```python
from build123d import *

# Parameters (mm, degrees)
EXTRUDE_THIN1_DEPTH = 165.1


with BuildPart() as part:
    # Sketch2 → Extrude-Thin1 (new body, symmetric)
    with BuildSketch(Plane(origin=(0, 0, 0), x_dir=(0, 0, -1), z_dir=(1, 0, 0))):
        with BuildLine():
            ThreePointArc((-60.240298086, -174.5682791), (-34.255387925, -150.550644745), (-24.65, -116.494825288))
            Line((-24.65, -116.494825288), (-24.65, -25.4))
            ThreePointArc((-24.65, -25.4), (-17.430182156, -7.969817844), (0, -0.75))
            Line((0, -0.75), (76.2, -0.75))
            Line((76.2, -0.75), (76.2, 0.75))
            Line((76.2, 0.75), (0, 0.75))
            ThreePointArc((0, 0.75), (-18.490842328, -6.909157672), (-26.15, -25.4))
            Line((-26.15, -25.4), (-26.15, -116.494825288))
            ThreePointArc((-26.15, -116.494825288), (-35.534320309, -149.766851432), (-60.921188809, -173.2317209))
            Line((-60.921188809, -173.2317209), (-60.240298086, -174.5682791))
        make_face()
    extrude(amount=EXTRUDE_THIN1_DEPTH, both=True)


solid = part.part
```
Design review of the part built by this model. Coordinates are the model's own, in mm. A direction names the side the tool comes from. Give positions to 0.01 mm unless a question says otherwise; leave off trailing zeros. Loops run counter-clockwise (first coordinate to the right, second up) from the corner with the lowest first, then second, coordinate; pieces in that order, holes last. Notation, with made-up numbers: (14.25, 46) -> (70.25, 46) arc R22 ccw to (70.25, 55) -> close; hole circle Ø1 at (18.5, -37). An arc over 180 degrees is marked (long way). Write each question's results on one line, items separated by ' | '.
Q1. Wall thickness on L1, parallel to Z at x = -93.5, y = -60.5; L2, parallel to Y at x = -37, z = -47.5: over which ranges is each line inside the solid? List them lowest first.
Reply:
L1: z = 24.65 to 26.15 | L2: y = -0.75 to 0.75
Q2. Take a section at A-A, the plane x = -15. Write out the cut boundary in (y, z) (3 decimals).
Reply:
outline: (-174.568, 60.24) arc R65.175 ccw to (-116.495, 24.65) -> (-25.4, 24.65) arc R24.65 cw to (-0.75, 0) -> (-0.75, -76.2) -> (0.75, -76.2) -> (0.75, 0) arc R26.15 ccw to (-25.4, 26.15) -> (-116.495, 26.15) arc R63.675 cw to (-173.232, 60.921) -> close
Q3. Take a section at B-B, the plane y = -50. Write out the cut boundary in (x, z), plus the area to 3 significant figures.
Reply:
outline: (-165.1, 24.65) -> (165.1, 24.65) -> (165.1, 26.15) -> (-165.1, 26.15) -> close | area: 495 mm²
Q4. For pin 1 Ø1 at (x, z) = (73, 43.5) entering from -Y; pin 2 Ø5 at (x, z) = (-25.5, 13.5) entering from -Y; pin 3 Ø8 at (x, y) = (116, -156.5) entering from -Z, all flat-tipped, find the tip position at first contact; note any pin that passes through.
Reply:
pin 1: stops at y = -162.84 | pin 2: stops at y = -6.65 | pin 3: stops at z = 35.5
Q5. Machinability: for faces 1 (the face through (2, 0.75, -39)), 2 (the face through (2, -70, 26.15)), 3 (the face through (2, -0.75, -38)), which of the approach directions +Z, -Z, +X, -X, +Y, -Y give a long, thin tool a straight path to every point of the face, cutting with its end or side? Answer none if there is none.
Reply:
face 1: +Z, -Z, +X, -X, +Y | face 2: +Z, +X, -X, +Y | face 3: -Z, +X, -X, -Y
Q6. Take a section at C-C, the plane z = -40. Write out the cut boundary in (x, y), plus the area to 3 significant figures.
Reply:
outline: (-165.1, -0.75) -> (165.1, -0.75) -> (165.1, 0.75) -> (-165.1, 0.75) -> close | area: 495 mm²
